CAD build for the part. Positions are in the model's coordinates, mm. Coordinates: 2 decimals unless noted, no trailing zeros. Loops run counter-clockwise (first coordinate to the right, second up) from the corner with the lowest first, then second, coordinate; pieces in that order, holes last. Notation, with made-up numbers: (-8.75, -31.5) -> (28.25, -31.5) arc R34 ccw to (28.25, 2.5) -> close; hole circle Ø7 at (44.5, -12). An arc over 180 degrees is marked (long way). Answer as a JSON object with one key per item and string values. Group by question number.
Autodesk Inventor part; units mm, degrees
ref_plane "YZ Plane" through (0, 0, 0) normal (1, 0, 0) x (0, 1, 0)
ref_plane "XZ Plane" through (0, 0, 0) normal (0, 1, 0) x (-1, 0, 0)
ref_plane "XY Plane" through (0, 0, 0) normal (0, 0, 1) x (1, 0, 0)
sketch "Sketch1" plane through (0, 0, 0) normal (0, 0, 1) x (1, 0, 0)
  circle A0 centre (29.8858, 59.5313) radius 2.3813
  circle A1 centre (-30.4392, 59.5313) radius 2.3812
  circle A2 centre (-30.4392, 91.2813) radius 2.3813
  circle A3 centre (29.8858, 91.2813) radius 2.3813
  circle A4 centre (-30.4392, 91.2813) radius 2.3813
  circle A5 centre (29.8858, 91.2813) radius 2.3813
  line L0 (-35.2017, 84.9313) -> (34.6483, 84.9313)
  line L1 (34.6483, 84.9313) -> (34.6483, 101.6)
  line L2 (34.6483, 101.6) -> (-35.2017, 101.6)
  line L3 (-35.2017, 101.6) -> (-35.2017, 84.9313)
  line L4 (34.6483, 101.6) -> (-35.2017, 101.6)
  line L5 (-35.2017, 101.6) -> (-35.2017, 50.8)
  line L6 (-35.2017, 50.8) -> (34.6483, 50.8)
  line L7 (34.6483, 50.8) -> (34.6483, 101.6)
  point P0 (0, 0)
  dimension "d0" = 50.8
extrude "Extrusion1" add sketch "Sketch1" along normal blind 15.875
sketch "Sketch2" plane through (-35.2017, 50.8, 0) normal (-1, 0, 0) x (0, 0, 1)
  arc A0 (0, 34.1313) -> (0, 15.0813) centre (0, 24.6063) ccw
  circle A1 centre (0, 24.6063) radius 9.525
  point P0 (0, -50.8)
  point P1 (0, 15.0813)
  point P2 (0, 34.1313)
extrude "Extrusion2" cut sketch "Sketch2" against normal blind 76.2
properties part number "YClampTop"
Item 1: Flat gauge pin, fed straight in: P1, Ø1.5, axis at x = 13.5, y = 68.5, coming from the -Z side. Where does the tip first touch, or does it go through?
Item 2: Band-saw the part on C-C, the plane z = 11.75. List the corners of the cut face in (x, y), and give its area (3 significant figures).
Item 3: Pull direction Y, two halves, no side cores. Call faces 1 (the flat face through (0, 101.6, 8)), 2 (the cylindrical face through (-0.766, 75.197, 9.523)), 3 (the flat face through (-1, 93, 0)), 4 (the flat face through (-1, 50.8, 8)): +Y half, -Y half, draft (parallel to the pull), parting line (faces both ways), or undercut.
Item 4: Band-saw the part on B-B, the plane x = -10.5. List the corners of the cut face in (y, z) (3 decimals), and give its area (3 significant figures).
Item 5: Band-saw the part on D-D, the plane y = 81. List the corners of the cut face in (x, z) (3 decimals), and give its area (3 significant figures).
Item 6: Drill centre lines: L1, parallel to X at y = 61.5, z = 6.25; L2, parallel to Y at x = -6, z = 3; L3, parallel to Y at x = 24.5, z = 2.75. Where is each one in solid material? Low to high.
Item 7: Band-saw the part on A-A, the plane z = 5. List the corners of the cut face in (x, y), and give its area (3 significant figures).
Reply:
{
 "1": {"P1": "z = 5.67"},
 "2": {"outline": "(-35.2, 50.8) -> (34.65, 50.8) -> (34.65, 101.6) -> (-35.2, 101.6) -> close; hole circle Ø4.76 at (-30.44, 59.53); hole circle Ø4.76 at (-30.44, 91.28); hole circle Ø4.76 at (29.89, 59.53); hole circle Ø4.76 at (29.89, 91.28)", "area": "3,480 mm²"},
 "3": {"face 1": "+Y half", "face 2": "undercut", "face 3": "draft", "face 4": "-Y half"},
 "4": {"outline": "(50.8, 0) -> (65.881, 0) arc R9.525 cw to (84.931, 0) -> (101.6, 0) -> (101.6, 15.875) -> (50.8, 15.875) -> close", "area": "664 mm²"},
 "5": {"outline": "(-35.202, 7.709) -> (34.648, 7.709) -> (34.648, 15.875) -> (-35.202, 15.875) -> close", "area": "570 mm²"},
 "6": {"L1": "-35.2 to -31.78, -29.1 to 28.55, 31.23 to 34.65", "L2": "50.8 to 66.37, 84.45 to 101.6", "L3": "50.8 to 66.29, 84.53 to 101.6"},
 "7": {"outline": "(-35.2, 50.8) -> (34.65, 50.8) -> (34.65, 67.3) -> (-35.2, 67.3) -> close; (-35.2, 83.51) -> (34.65, 83.51) -> (34.65, 101.6) -> (-35.2, 101.6) -> close; hole circle Ø4.76 at (-30.44, 59.53); hole circle Ø4.76 at (-30.44, 91.28); hole circle Ø4.76 at (29.89, 59.53); hole circle Ø4.76 at (29.89, 91.28)", "area": "2,340 mm²"}
}
